Can you work these out from the drawing? Everything is in mm from the part's minimum corner. Round coordinates to 2 decimals unless told otherwise and drop trailing zeros. Write each loop counter-clockwise with the first axis right and the second up, starting at its lowest first coordinate (ties: lowest second). Pieces come first, ordered by that corner, then holes. Notation, with made-up numbers: (71.25, -21) - (86.25, -21) arc R23 ccw to (86.25, 16) - close; hole circle Ø2 at (14.5, 30.5). An arc over 180 degrees is marked (long way). Write each question's results on one line, items separated by ' | '. Start each with the question number.
(1) Imagine slicing it at B-B on y = 48.5. Write out the boundary of the cut face in (x, z), then the cut area to 3 significant figures.
(2) Please list where these lines run through material, in increasing order: line 1 (Y direction, x = 125, z = 2.5); line 2 (X direction, y = 58.5, z = 4.5); line 3 (X direction, y = 40.5, z = 2.75). Write a range as [from, to].
(3) For P1, Ø1.5, axis at x = 88.5, z = 1, coming from the +Y side, with a flat end and sliding along its axis, tell me the tip position at first contact or that it passes through.
(4) Imagine slicing it at A-A on z = 3.5. Write out the boundary of the cut face in (x, y).
(5) Imagine slicing it at D-D on x = 116. Write out the boundary of the cut face in (y, z), then the cut area to 3 significant figures.
(6) Imagine slicing it at C-C on y = 59. Write out the boundary of the cut face in (x, z).
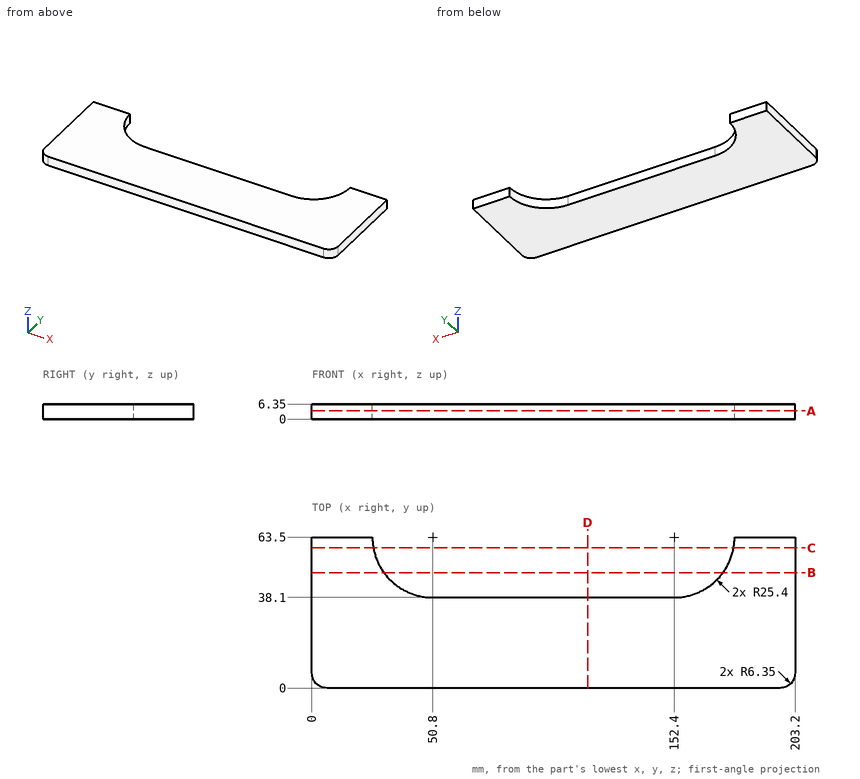
Response:
1) outline: (0, 0) - (30.3, 0) - (30.3, 6.35) - (0, 6.35) - close; (172.9, 0) - (203.2, 0) - (203.2, 6.35) - (172.9, 6.35) - close | area: 385 mm²
2) line 1: [0, 38.1] | line 2: [0, 25.9], [177.3, 203.2] | line 3: [0, 40.02], [163.18, 203.2]
3) P1: y = 38.1
4) outline: (0, 6.35) arc R6.35 ccw to (6.35, 0) - (196.85, 0) arc R6.35 ccw to (203.2, 6.35) - (203.2, 63.5) - (177.8, 63.5) arc R25.4 cw to (152.4, 38.1) - (50.8, 38.1) arc R25.4 cw to (25.4, 63.5) - (0, 63.5) - close
5) outline: (0, 0) - (38.1, 0) - (38.1, 6.35) - (0, 6.35) - close | area: 242 mm²
6) outline: (0, 0) - (25.8, 0) - (25.8, 6.35) - (0, 6.35) - close; (177.4, 0) - (203.2, 0) - (203.2, 6.35) - (177.4, 6.35) - close
